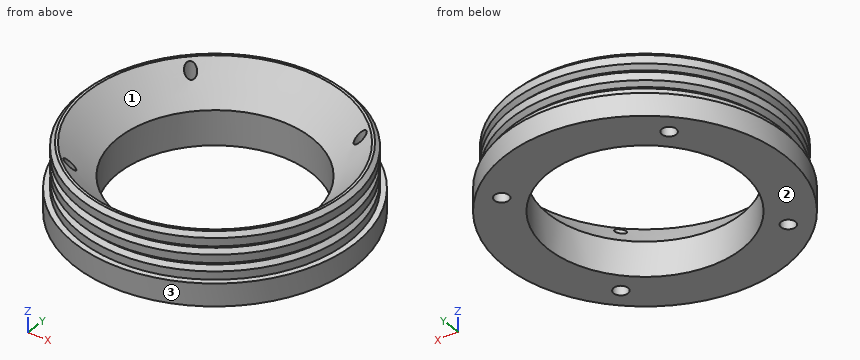
```python
from build123d import *

# Parameters (mm, degrees)
SKETCH2_R                  = 39.624
SKETCH2_R_2                = 27.3304
BOSS_EXTRUDE2_DEPTH        = 6.35
SKETCH5_R                  = 38.018820021
SKETCH5_R_2                = 27.3304
BOSS_EXTRUDE3_DEPTH        = 19.05
F_10_32_TAPPED_HOLE1_D     = 4.0386
F_10_32_TAPPED_HOLE1_DEPTH = 12.7
F_10_32_TAPPED_HOLE1_TIP   = 1.213317848
CUT_EXTRUDE2_DEPTH         = 60.186360354
CUT_EXTRUDE2_DEPTH_BACK    = 60.186360354
SKETCH16_R                 = 1.524


with BuildPart() as part:
    # Sketch2 → Boss-Extrude2 (new body)
    with BuildSketch(Plane.XY):
        Circle(SKETCH2_R)
        Circle(SKETCH2_R_2, mode=Mode.SUBTRACT)
    extrude(amount=BOSS_EXTRUDE2_DEPTH)

    # Sketch5 → Boss-Extrude3 (add)
    with BuildSketch(Plane.XY):
        with Locations(Location((0, 0, 0), (0, 0, 180))):
            Circle(SKETCH5_R)
        Circle(SKETCH5_R_2, mode=Mode.SUBTRACT)
    extrude(amount=BOSS_EXTRUDE3_DEPTH)

    # Sketch10 → Cut-Revolve2 (revolve, cut)
    with BuildSketch(Plane(origin=(0, 0, 0), x_dir=(0, 0, -1), z_dir=(1, 0, 0)), mode=Mode.PRIVATE) as cut_revolve2_sk:
        Polygon((-29.4386, 38.018820021), (-27.1272, 38.018820021), (-28.2829, 36.863120021), align=None)
        Polygon((-24.8158, 38.018820021), (-22.5044, 38.018820021), (-23.6601, 36.863120021), align=None)
        Polygon((-20.193, 38.018820021), (-17.8816, 38.018820021), (-19.0373, 36.863120021), align=None)
        Polygon((-15.5702, 38.018820021), (-13.2588, 38.018820021), (-14.4145, 36.863120021), align=None)
        Polygon((-10.9474, 38.018820021), (-8.636, 38.018820021), (-9.7917, 36.863120021), align=None)
    revolve(cut_revolve2_sk.sketch.rotate(Axis((0, 0, 50.084179241), (0, 0, 1)), 90), axis=Axis((0, 0, 50.084179241), (0, 0, 1)), mode=Mode.SUBTRACT)

    # Sketch11 → Cut-Revolve3 (revolve, cut)
    with BuildSketch(Plane(origin=(0, 0, 0), x_dir=(0, 0, -1), z_dir=(1, 0, 0)), mode=Mode.PRIVATE) as cut_revolve3_sk:
        Polygon((-19.685, 36.788548166), (-6.35, 24.088548166), (-19.685, 24.088548166), align=None)
    revolve(cut_revolve3_sk.sketch.rotate(Axis((0, 0, 43.100386529), (0, 0, 1)), 270), axis=Axis((0, 0, 43.100386529), (0, 0, 1)), mode=Mode.SUBTRACT)

    # 10-32 Tapped Hole1
    with Locations(Plane(origin=(0, 0, 0), x_dir=(1, 0, 0), z_dir=(0, 0, -1))):
        with Locations((23.671955135, 23.671955135), (0, 0), (23.671955135, -23.671955135), (-23.671955135, 23.671955135), (-23.671955135, -23.671955135)):
            Hole(F_10_32_TAPPED_HOLE1_D / 2, depth=F_10_32_TAPPED_HOLE1_DEPTH)
            with Locations((0, 0, -(F_10_32_TAPPED_HOLE1_DEPTH + F_10_32_TAPPED_HOLE1_TIP / 2))):  # 118° drill point
                Cone(0, F_10_32_TAPPED_HOLE1_D / 2, F_10_32_TAPPED_HOLE1_TIP, mode=Mode.SUBTRACT)

    # Sketch16 → Cut-Extrude2 (cut, two sides: drawn at the far end of the back side and taken through both)
    with BuildSketch(Plane(origin=(0, 0, 0), x_dir=(-1, 0, 0), z_dir=(0, 0, -1)).offset(-CUT_EXTRUDE2_DEPTH_BACK)):
        with Locations(Location((23.977283843, 23.977283843, 0), (0, 0, 225))):
            Circle(SKETCH16_R)
        with Locations(Location((-23.977283843, 23.977283843, 0), (0, 0, 305.409590833))):
            Circle(SKETCH16_R)
        with Locations(Location((-23.977283843, -23.977283843, 0), (0, 0, 305.973376129))):
            Circle(SKETCH16_R)
        with Locations(Location((23.977283843, -23.977283843, 0), (0, 0, 135))):
            Circle(SKETCH16_R)
    extrude(amount=CUT_EXTRUDE2_DEPTH + CUT_EXTRUDE2_DEPTH_BACK, mode=Mode.SUBTRACT)


solid = part.part
```
The listing builds one solid part. Answer for the finished solid, in the listing's coordinates (mm). Face numbers are marked on the shaded views. Coordinates: 2 decimals unless noted, no trailing zeros. Loops run counter-clockwise (first coordinate to the right, second up) from the corner with the lowest first, then second, coordinate; pieces in that order, holes last. Notation, with made-up numbers: (24, 30) -> (64, 30) arc R37 cw to (64, 66) -> close; hole circle Ø4 at (50.5, -13). An arc over 180 degrees is marked (long way). Return JSON: item names as keys, results as strings. Group by question number.
(1) Determine the mould class of the marked faces 1, 2 and 3 for opening direction Y: released by +Y, released by -Y, zero draft, split by the parting line, or undercut.
(2) A cutting plane is placed at C-C on z = 3.5. Write down the section's boundary in (x, y).
(3) Find the intervals of material crossed by probe 1 along X at (y, z) = (11.5, 13); probe 2 along Y at (x, z) = (-5.5, 6.75); probe 3 along X at (y, z) = (23, 10.75), in increasing order. Write a range as from..to.
(4) Given pin 1 Ø3.5 at (x, y) = (-23.67, -23.67) entering from -Z; pin 2 Ø2 at (x, z) = (5.5, 9.5) entering from -Y; pin 3 Ø3 at (x, y) = (-23.67, 23.67) entering from -Z, each flat-ended and moving along its own axis, determine where each tip first touches the part or whether it passes through.
The answers:
{
 "1": {"face 1": "undercut", "face 2": "zero draft", "face 3": "split by the parting line"},
 "2": {"outline": "circle Ø79.25 at (0, 0); hole circle Ø54.66 at (0, 0); hole circle Ø4.04 at (-23.67, -23.67); hole circle Ø4.04 at (-23.67, 23.67); hole circle Ø4.04 at (23.67, -23.67); hole circle Ø4.04 at (23.67, 23.67)"},
 "3": {"probe 1": "x = -36.24..-28.16, 28.16..36.24", "probe 2": "y = -37.62..-26.77, 26.77..37.62", "probe 3": "x = -30.02..-25.58, -21.77..-16.45, 16.45..21.77, 25.58..30.02"},
 "4": {"pin 1": "stops at z = 12.86", "pin 2": "stops at y = -37.69", "pin 3": "stops at z = 13.01"}
}
